Geometry check sheet. Reference: the model listing, model coordinates, mm. A direction names the side the tool comes from. Coordinates: 2 decimals unless noted, no trailing zeros. Loops run counter-clockwise (first coordinate to the right, second up) from the corner with the lowest first, then second, coordinate; pieces in that order, holes last.
from build123d import *

# Parameters (mm, degrees)
F0_R          = 3.81
F1_DEPTH      = 12.7
F1_DEPTH_BACK = 50.8
F2_W          = 64.77
F2_H          = 10.16
F2_W_2        = 10.16
F2_H_2        = 64.77
F3_DEPTH      = 3.81
F4_SIZE2      = 4.540571
F4_SIZE       = 3.80999
F4_2_SIZE2    = 4.540571
F4_2_SIZE     = 3.80999
F4_3_SIZE2    = 4.540571
F4_3_SIZE     = 3.80999
F4_4_SIZE2    = 4.540571
F4_4_SIZE     = 3.80999


# Not quite as in the source:
# - a fillet or chamfer is up to 0.001 mm smaller than in the source, because OpenCascade refuses the exact size


with BuildPart() as f1:
    # F0 (on Right) → F1 (new body, two sides)
    with BuildSketch(Plane.YZ) as f1_sk:
        Circle(F0_R)
    extrude(amount=F1_DEPTH)
    extrude(f1_sk.sketch, amount=-F1_DEPTH_BACK)

    # F2 (on face) → F3 (join)
    with BuildSketch(Plane.YZ.offset(12.7)):
        with Locations((37.465, 0)):
            Rectangle(F2_W, F2_H)
        Rectangle(F2_W_2, F2_H)
        with Locations((0, 37.465)):
            Rectangle(F2_W_2, F2_H_2)
        with Locations((-37.465, 0)):
            Rectangle(F2_W, F2_H)
        with Locations((0, -37.465)):
            Rectangle(F2_W_2, F2_H_2)
    extrude(amount=F3_DEPTH)

    # F4 (size 3.81 and 4.5405811878 in the source; OpenCascade refuses exactly that, so slightly less here)
    f4_edges = [f1.edges().sort_by_distance(p)[0] for p in [
        (16.51, 5.08, 37.465),
    ]]
    f4_side = f1.faces().sort_by_distance((14.605, 5.08, 37.465))[0]
    chamfer(f4_edges, length=F4_SIZE, length2=F4_SIZE2, reference=f4_side)

    # F4#2 (size 3.81 and 4.5405811878 in the source; OpenCascade refuses exactly that, so slightly less here)
    f4_2_edges = [f1.edges().sort_by_distance(p)[0] for p in [
        (16.51, 37.465, -5.08),
    ]]
    f4_2_side = f1.faces().sort_by_distance((14.605, 37.465, -5.08))[0]
    chamfer(f4_2_edges, length=F4_2_SIZE, length2=F4_2_SIZE2, reference=f4_2_side)

    # F4#3 (size 3.81 and 4.5405811878 in the source; OpenCascade refuses exactly that, so slightly less here)
    f4_3_edges = [f1.edges().sort_by_distance(p)[0] for p in [
        (16.51, -5.08, -37.465),
    ]]
    f4_3_side = f1.faces().sort_by_distance((14.605, -5.08, -37.465))[0]
    chamfer(f4_3_edges, length=F4_3_SIZE, length2=F4_3_SIZE2, reference=f4_3_side)

    # F4#4 (size 3.81 and 4.5405811878 in the source; OpenCascade refuses exactly that, so slightly less here)
    f4_4_edges = [f1.edges().sort_by_distance(p)[0] for p in [
        (16.51, -37.465, 5.08),
    ]]
    f4_4_side = f1.faces().sort_by_distance((14.605, -37.465, 5.08))[0]
    chamfer(f4_4_edges, length=F4_4_SIZE, length2=F4_4_SIZE2, reference=f4_4_side)


solid = f1.part
1) Section check B-B on x = -25.5. Record the cut outline in (y, z), and give its area (3 significant figures).
Data:
outline: circle Ø7.62 at (0, 0)
area: 45.6 mm2
2) Access from +Z, -Z, +X, -X, +Y, -Y to the whole of each face (thin tool, end or side, straight path). Record for faces 1 (the flat face through (14.63, 37.01, -2.78)), 2 (the flat face through (14.63, 2.78, 37.01)), 3 (the cylindrical face through (-18.61, -0.83, -3.72)), 4 (the flat face through (14.63, -2.78, -37.92)).
Data:
face 1: -Z, +X, +Y
face 2: +Z, +X, +Y
face 3: -X
face 4: -Z, +X, -Y
3) Depth check by flat-ended pin: pin 1 (3 mm diameter, centred on x = 15.5, y = -26, fed in from -Z); pin 2 (10 mm diameter, centred on x = -31.5, z = 8.5, fed in from -Y); pin 3 (1.9 mm diameter, centred on x = 15.5, z = -35, fed in from +Y); pin 4 (5 mm diameter, centred on y = 8.5, z = 48, fed in from -X). Enter the tip coordinate at first touch or a pass-through.
Data:
pin 1: stops at z = -5.08
pin 2: stops at y = -1.51
pin 3: stops at y = 5.08
pin 4: passes through
4) Material ranges on probe 1 along X at (y, z) = (-41, -5); probe 2 along Z at (x, y) = (-48, 1), recorded low to high.
Data:
probe 1: x = 12.7 to 16.51
probe 2: z = -3.68 to 3.68
